```python
from build123d import *

# Parameters (mm, degrees)
F0_W      = 107.95
F0_H      = 400.05
F1_DEPTH  = 6.35
F2_W      = 107.95
F2_H      = 6.35
F3_DEPTH  = 533.4
F4_W      = 6.35
F4_H      = 387.35
F5_DEPTH  = 533.4
F6_W      = 107.95
F6_H      = 400.05
F7_DEPTH  = 6.35
F9_DEPTH  = 387.35
F11_DEPTH = 387.35


with BuildPart() as f1:
    # F0 (on Top) → F1 (new body)
    with BuildSketch(Plane.XY):
        with Locations((53.975, 200.025)):
            Rectangle(F0_W, F0_H)
    extrude(amount=F1_DEPTH)

    # F2 (on face) → F3 (join)
    with BuildSketch(Plane.XY.offset(6.35)):
        with Locations((53.975, 3.175)):
            Rectangle(F2_W, F2_H)
        with Locations((53.975, 396.875)):
            Rectangle(F2_W, F2_H)
    extrude(amount=F3_DEPTH)

    # F4 (on face) → F5 (join)
    with BuildSketch(Plane.XY.offset(6.35)):
        with Locations((3.175, 200.025)):
            Rectangle(F4_W, F4_H)
    extrude(amount=F5_DEPTH)

    # F6 (on face) → F7 (join)
    with BuildSketch(Plane.XY.offset(539.75)):
        with Locations((53.975, 200.025)):
            Rectangle(F6_W, F6_H)
    extrude(amount=F7_DEPTH)

    # F8 (on face) → F9 (join)
    with BuildSketch(Plane(origin=(0, 6.35, 0), x_dir=(-1, 0, 0), z_dir=(0, 1, 0))):
        Polygon((-18.566158, 0), (0, 0), (-107.95, 39.290587), (-107.95, 32.533058), align=None)
    extrude(amount=F9_DEPTH)

    # F10 (on face) → F11 (join)
    with BuildSketch(Plane(origin=(0, 6.35, 0), x_dir=(-1, 0, 0), z_dir=(0, 1, 0))):
        Polygon((-107.95, 134.948116), (-107.95, 128.190587), (-6.35, 91.211211), (-6.35, 97.96874), align=None)
    extrude(amount=F11_DEPTH)


solid = f1.part
```
Here's how the part is built. I have some questions about the finished solid (model axes, mm). A direction names the side the tool comes from. Coordinates: 2 decimals unless noted, no trailing zeros. Order: outer loops, then holes, each group sorted by start corner. A loop starts at its lowest first (then second) coordinate and runs counter-clockwise, first axis right, second up. Notation, with made-up numbers: M 66,-2 L 92,-2 A8 ccw 92,3 Z; hole C -9.75,-30.75 d8. An arc over 180 degrees is marked long. Answer as a JSON object with one key per item and string values. Group by question number.
(1) Suppose I cut it at C-C, the plane z = 420. Please give me the cut outline in (x, y).
(2) For pin 1 (1 mm diameter, centred on y = 239, z = 294, fed in from +X), with a flat end and sliding along its axis, tell me the tip position at first contact or that it passes through.
(3) I need wall thicknesses on probe 1 along Y at (x, z) = (10.5, 435); probe 2 along Z at (x, y) = (74, 242.5); probe 3 along Z at (x, y) = (13, 182). Which ranges of each line are inside material? Lowest first, please.
(4) Suppose I cut it at D-D, the plane x = 23. Please give me the cut outline in (y, z).
(5) If we mould it in two halves opening along Z, with no side actions, what happens to faces 4 (the face through (55, 197, 0)), 5 (the face through (53, 203, 546.1)), 6 (the face through (57.86, 197.31, 109.96))? For each: released by +Z, released by -Z, zero draft, split by the parting line, or undercut.
(6) Which directions (+Z, -Z, +X, -X, +Y, -Y) give clear straight access to the entire face, cutting with the end or side of a thin tool? Please do faces 1 (the face through (53, 400.05, 269)), 2 (the face through (56, 6.35, 66)), 3 (the face through (87, 393.7, 13)).
(7) Suppose I cut it at A-A, the plane y = 366. Please give me the cut outline in (x, z).
(8) Suppose I cut it at B-B, the plane x = 62. Please give me the cut outline in (y, z), then the cut area to 3 significant figures.
Values found:
{
 "1": {"outline": "M 0,0 L 107.95,0 L 107.95,6.35 L 6.35,6.35 L 6.35,393.7 L 107.95,393.7 L 107.95,400.05 L 0,400.05 Z"},
 "2": {"pin 1": "stops at x = 6.35"},
 "3": {"probe 1": "y = 0 to 6.35, 393.7 to 400.05", "probe 2": "z = 0 to 6.35, 20.18 to 26.93, 115.83 to 122.59, 539.75 to 546.1", "probe 3": "z = 0 to 6.35, 93.63 to 100.39, 539.75 to 546.1"},
 "4": {"outline": "M 0,0 L 400.05,0 L 400.05,546.1 L 0,546.1 Z; hole M 6.35,8.37 L 393.7,8.37 L 393.7,97.27 L 6.35,97.27 Z; hole M 6.35,104.03 L 393.7,104.03 L 393.7,539.75 L 6.35,539.75 Z"},
 "5": {"face 4": "released by -Z", "face 5": "released by +Z", "face 6": "undercut"},
 "6": {"face 1": "+Z, -Z, +X, -X, +Y", "face 2": "none", "face 3": "+X"},
 "7": {"outline": "M 0,0 L 107.95,0 L 107.95,6.35 L 36.01,6.35 L 107.95,32.53 L 107.95,39.29 L 17.45,6.35 L 6.35,6.35 L 6.35,91.21 L 107.95,128.19 L 107.95,134.95 L 6.35,97.97 L 6.35,539.75 L 107.95,539.75 L 107.95,546.1 L 0,546.1 Z"},
 "8": {"outline": "M 0,0 L 400.05,0 L 400.05,546.1 L 0,546.1 Z; hole M 6.35,6.35 L 393.7,6.35 L 393.7,15.81 L 6.35,15.81 Z; hole M 6.35,22.57 L 393.7,22.57 L 393.7,111.47 L 6.35,111.47 Z; hole M 6.35,118.22 L 393.7,118.22 L 393.7,539.75 L 6.35,539.75 Z", "area": "17,100 mm^2"}
}
